Could you check a few things on this model? Use its own coordinates, in mm. Face numbers are marked on the shaded views. A direction names the side the tool comes from. Round coordinates to 2 decimals unless told otherwise and drop trailing zeros. Loops run counter-clockwise (first coordinate to the right, second up) from the corner with the lowest first, then second, coordinate; pieces in that order, holes last. Notation, with made-up numbers: (-27, -8.5) - (-1, -8.5) arc R27 cw to (-1, 15.5) - close; hole circle Ø6 at (53.25, 35.25). An arc over 180 degrees is marked (long way). Put each result on its own line as item: value. Start each with the question number.
from build123d import *

# Parameters (mm, degrees)
SKETCH2_W               = 100
SKETCH2_H               = 3
BOSS_EXTRUDE1_DEPTH     = 22
SKETCH3_R               = 2.5
BOSS_EXTRUDE2_DEPTH     = 10
SKETCH4_R               = 1.5
BOSS_EXTRUDE3_DEPTH     = 15
CUT_EXTRUDE1_DEPTH      = 81.991511901
CUT_EXTRUDE1_DEPTH_BACK = 81.991511901


with BuildPart() as part:
    # Sketch2 → Boss-Extrude1 (new body)
    with BuildSketch(Plane(origin=(0, 0, 0), x_dir=(1, 0, 0), z_dir=(0, 1, 0))):
        Rectangle(SKETCH2_W, SKETCH2_H)
    extrude(amount=BOSS_EXTRUDE1_DEPTH)

    # Sketch3 → Boss-Extrude2 (add)
    with BuildSketch(Plane(origin=(0, 22, 0), x_dir=(1, 0, 0), z_dir=(0, 1, 0))):
        with BuildLine():
            Line((50, 1.5), (-58.563068229, 1.5))
            ThreePointArc((-58.563068229, 1.5), (-65.75, 0), (-58.563068229, -1.5))
            Line((-58.563068229, -1.5), (50, -1.5))
            Line((50, -1.5), (50, 1.5))
        make_face()
        with Locations(Location((-62, 0, 0), (0, 0, 270))):
            Circle(SKETCH3_R, mode=Mode.SUBTRACT)
    extrude(amount=BOSS_EXTRUDE2_DEPTH)

    # Sketch4 → Boss-Extrude3 (add)
    with BuildSketch(Plane(origin=(0, 32, 0), x_dir=(1, 0, 0), z_dir=(0, 1, 0))):
        with Locations(Location((-46, 0, 0), (0, 0, 270))):
            Circle(SKETCH4_R)
    extrude(amount=BOSS_EXTRUDE3_DEPTH)

    # Sketch5 → Cut-Extrude1 (cut, two sides: drawn at the far end of the back side and taken through both)
    with BuildSketch(Plane.XY.offset(1.5).offset(-CUT_EXTRUDE1_DEPTH_BACK)):
        Polygon((-65.75, 27), (-65.75, 24.25), (-50, 24.25), (-50, 29.75), (-65.75, 29.75), align=None)
    extrude(amount=CUT_EXTRUDE1_DEPTH + CUT_EXTRUDE1_DEPTH_BACK, mode=Mode.SUBTRACT)


solid = part.part
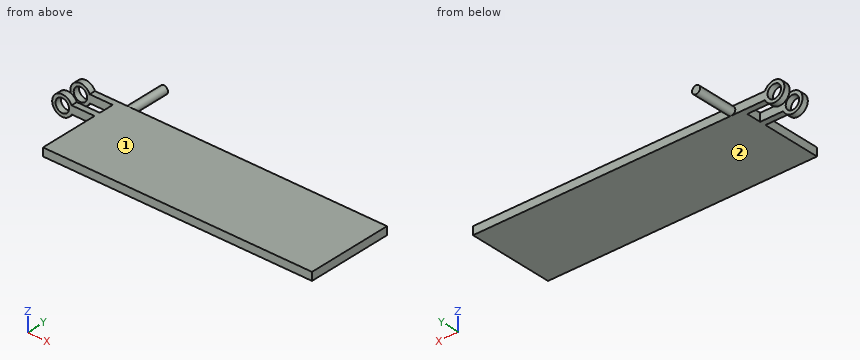
Item 1: Suppose I cut it at C-C, the plane y = 39. List the corners of the cut face in (x, z) for me, then the cut area to 3 significant figures.
Item 2: Will these pins go through, and if not, where does the flat tip stop? P1, Ø2, axis at x = -52.5, z = 2, coming from the +Y side; P2, Ø9.5, axis at x = -17.5, y = 19.5, coming from the +Z side; P3, Ø3.5, axis at y = 26.5, z = 0.5, coming from the -X side.
Item 3: Suppose I cut it at A-A, the plane x = -56. List the corners of the cut face in (y, z) for me, then the cut area to 3 significant figures.
Item 4: Suppose I cut it at B-B, the plane z = 0. List the corners of the cut face in (x, y) for me, then the cut area to 3 significant figures.
Item 5: On a 3-axis mill with a long thin cutter (end or side, diameter ignored), from which of +Z, -Z, +X, -X, +Y, -Y can I reach the whole of each face in a straight line? I mean the marked faces 1 and 2. Say none if no direction works.
Item 6: Suppose I cut it at D-D, the plane x = 41. List the corners of the cut face in (y, z) for me.
Item 7: I need wall thicknesses on line 1 (Z direction, x = -62, y = 23); line 2 (X direction, y = 22.75, z = 0); line 3 (Y direction, x = -56, z = -0.75). Which ranges of each line are inside material? Lowest first, please. Write a range as from..to.
Numbers:
1. outline: circle Ø3 at (-46, 0)
1. area: 7.07 mm^2
2. P1: y = 32
2. P2: z = 1.5
2. P3: x = -50
3. outline: (22, -1.5) - (24.25, -1.5) - (24.25, 1.5) - (22, 1.5) - close; (29.75, -1.5) - (32, -1.5) - (32, 1.5) - (29.75, 1.5) - close
3. area: 13.5 mm^2
4. outline: (-65.75, 22) - (-64.5, 22) - (-64.5, 24.25) - (-65.75, 24.25) - close; (-65.75, 29.75) - (-64.5, 29.75) - (-64.5, 32) - (-65.75, 32) - close; (-59.5, 22) - (-50, 22) - (-50, 0) - (50, 0) - (50, 32) - (-44.5, 32) - (-44.5, 47) - (-47.5, 47) - (-47.5, 32) - (-59.5, 32) - (-59.5, 29.75) - (-50, 29.75) - (-50, 24.25) - (-59.5, 24.25) - close
4. area: 3,290 mm^2
5. face 1: +Z, +X, +Y, -Y
5. face 2: -Z, +X, +Y, -Y
6. outline: (0, -1.5) - (32, -1.5) - (32, 1.5) - (0, 1.5) - close
7. line 1: -3.75..-2.5, 2.5..3.75
7. line 2: -65.75..-64.5, -59.5..50
7. line 3: 22..24.25, 29.75..32
